Input: part model. Units: mm. Frame: model coordinates. Give positions to 0.01 mm unless a question says otherwise; leave off trailing zeros. Loops run counter-clockwise (first coordinate to the right, second up) from the corner with the lowest first, then second, coordinate; pieces in that order, holes last. Notation, with made-up numbers: M 3,-19 L 42,-19 A26 ccw 42,3 Z; hole C -4.75,67 d9. An arc over 180 degrees is marked long. Return JSON: item names as keys, results as strings. Group by question number.
```python
from build123d import *

# Parameters (mm, degrees)
SKETCH_1_R          = 2
EXTRUDE_1_DEPTH     = 4
CUT_EXTRUDE_1_DEPTH = 4
EXTRUDE_2_DEPTH     = 4
EXTRUDE_3_DEPTH     = 4
SKETCH_18_R         = 2
CUT_EXTRUDE_2_DEPTH = 5
CUT_EXTRUDE_3_DEPTH = 5


with BuildPart() as part:
    # 草图1 → 凸台-拉伸1 (new body)
    with BuildSketch(Plane.XY):
        with BuildLine():
            Line((153.5, -28), (-153.5, -28))
            ThreePointArc((-153.5, -28), (-156.328427125, -26.828427125), (-157.5, -24))
            Line((-157.5, -24), (-157.5, 24))
            ThreePointArc((-157.5, 24), (-156.328427125, 26.828427125), (-153.5, 28))
            Line((-153.5, 28), (153.5, 28))
            ThreePointArc((153.5, 28), (156.328427125, 26.828427125), (157.5, 24))
            Line((157.5, 24), (157.5, -24))
            ThreePointArc((157.5, -24), (156.328427125, -26.828427125), (153.5, -28))
        make_face()
        with Locations((-100, 23)):
            Circle(SKETCH_1_R, mode=Mode.SUBTRACT)
        with Locations((-61.67, 23)):
            Circle(SKETCH_1_R, mode=Mode.SUBTRACT)
        with Locations((-100, -23)):
            Circle(SKETCH_1_R, mode=Mode.SUBTRACT)
        with Locations((-61.67, -23)):
            Circle(SKETCH_1_R, mode=Mode.SUBTRACT)
        with Locations((100, -23)):
            Circle(SKETCH_1_R, mode=Mode.SUBTRACT)
        with Locations((61.67, -23)):
            Circle(SKETCH_1_R, mode=Mode.SUBTRACT)
        with Locations((61.67, 23)):
            Circle(SKETCH_1_R, mode=Mode.SUBTRACT)
        with Locations((100, 23)):
            Circle(SKETCH_1_R, mode=Mode.SUBTRACT)
        with BuildLine():
            Line((-150, -13.9), (-50, -13.9))
            ThreePointArc((-50, -13.9), (-47.9, -16), (-50, -18.1))
            Line((-50, -18.1), (-150, -18.1))
            ThreePointArc((-150, -18.1), (-152.1, -16), (-150, -13.9))
        make_face(mode=Mode.SUBTRACT)
    extrude(amount=EXTRUDE_1_DEPTH)

    # 草图2 → 切除-拉伸1 (cut)
    with BuildSketch(Plane.XY.offset(4)):
        with BuildLine():
            Line((0, -12), (0, -24))
            ThreePointArc((0, -24), (-1.171572875, -26.828427125), (-4, -28))
            Line((-4, -28), (0, -28))
            Line((0, -28), (157.5, -28))
            Line((157.5, -28), (157.5, -2))
            Line((157.5, -2), (157.5, 2))
            ThreePointArc((157.5, 2), (156.328427125, -0.828427125), (153.5, -2))
            Line((153.5, -2), (146.462792112, -2))
            Line((146.462792112, -2), (108, -2))
            Line((108, -2), (10, -2))
            ThreePointArc((10, -2), (2.928932188, -4.928932188), (0, -12))
        make_face()
    extrude(amount=-CUT_EXTRUDE_1_DEPTH, mode=Mode.SUBTRACT)

    # 草图3 → 凸台-拉伸2 (add)
    with BuildSketch(Plane.XY.offset(4)):
        with BuildLine():
            Line((-4, 28), (-4, -28))
            ThreePointArc((-4, -28), (-1.171572875, -26.828427125), (0, -24))
            Line((0, -24), (0, -12))
            ThreePointArc((0, -12), (2.928932188, -4.928932188), (10, -2))
            Line((10, -2), (26, -2))
            Line((26, -2), (26, 24))
            ThreePointArc((26, 24), (27.171572875, 26.828427125), (30, 28))
            Line((30, 28), (26, 28))
            Line((26, 28), (-4, 28))
        make_face()
        with BuildLine():
            ThreePointArc((0, -24), (-1.171572875, -26.828427125), (-4, -28))
            Line((-4, -28), (22, -28))
            ThreePointArc((22, -28), (24.828427125, -26.828427125), (26, -24))
            Line((26, -24), (26, -2))
            Line((26, -2), (10, -2))
            ThreePointArc((10, -2), (2.928932188, -4.928932188), (0, -12))
            Line((0, -12), (0, -24))
        make_face()
    extrude(amount=-EXTRUDE_2_DEPTH)

    # 草图17 → 凸台-拉伸3 (add)
    with BuildSketch(Plane.XY.offset(4)):
        with BuildLine():
            Line((26, -2), (26, -8.742458912))
            Line((26, -8.742458912), (26, -17))
            ThreePointArc((26, -17), (30.393398282, -6.393398282), (41, -2))
            Line((41, -2), (26, -2))
        make_face()
    extrude(amount=-EXTRUDE_3_DEPTH)

    # 草图18 → 切除-拉伸2 (cut, through all)
    with BuildSketch(Plane.XY.offset(4)):
        with Locations((0, -16)):
            Circle(SKETCH_18_R)
    extrude(amount=-CUT_EXTRUDE_2_DEPTH, mode=Mode.SUBTRACT)

    # 草图19 → 切除-拉伸3 (cut, through all)
    with BuildSketch(Plane.XY.offset(4)):
        with BuildLine():
            Line((-50, -10.6), (-150, -10.6))
            ThreePointArc((-150, -10.6), (-153.6, -7), (-150, -3.4))
            Line((-150, -3.4), (-50, -3.4))
            ThreePointArc((-50, -3.4), (-46.4, -7), (-50, -10.6))
        make_face()
    extrude(amount=-CUT_EXTRUDE_3_DEPTH, mode=Mode.SUBTRACT)


solid = part.part
```
Item 1: Section D-D, the plane x = 74.5. Return loops of the section in (y, z), then the cut area to 3 significant figures.
Item 2: Material intervals for line 1 (Y direction, x = -61.67, z = 0.9); line 2 (Y direction, x = -143, z = 2.9); line 3 (X direction, y = -15.5, z = 0.85), sorted ascending. Write a range as from..to.
Item 3: First-contact query: pin 1 Ø2 at (y, z) = (-21, 2) entering from +X; pin 2 Ø8 at (x, y) = (-124.5, 16.5) entering from -Z; pin 3 Ø1.5 at (y, z) = (-15, 0.5) entering from +X; pin 4 Ø2.5 at (x, y) = (-100, 23) entering from +Z. Flat tips, straight axial feed; report the tip coordinate or a pass-through.
Item 4: Section C-C, the plane y = -7. Return loops of the section in (x, z).
Item 5: Section A-A, the plane x = -114. Return loops of the section in (y, z), then the cut area to 3 significant figures.
Item 6: Section B-B, the plane z = 2.3. Give the number of separate pieces and of enclosed holes in the cut face, then the cut area to 3 significant figures.
Answer below:
{
 "1": {"outline": "M -2,0 L 28,0 L 28,4 L -2,4 Z", "area": "120 mm^2"},
 "2": {"line 1": "-28..-25, -21..-18.1, -13.9..-10.6, -3.4..21, 25..28", "line 2": "-28..-18.1, -13.9..-10.6, -3.4..28", "line 3": "-157.5..-152.04, -47.96..-1.94, 1.94..26.08"},
 "3": {"pin 1": "x = 26", "pin 2": "z = 0", "pin 3": "x = 26.25", "pin 4": "through"},
 "4": {"outline": "M -157.5,0 L -153.6,0 L -153.6,4 L -157.5,4 Z; M -46.4,0 L 29.82,0 L 29.82,4 L -46.4,4 Z"},
 "5": {"outline": "M -28,0 L -18.1,0 L -18.1,4 L -28,4 Z; M -13.9,0 L -10.6,0 L -10.6,4 L -13.9,4 Z; M -3.4,0 L 28,0 L 28,4 L -3.4,4 Z", "area": "178 mm^2"},
 "6": {"separate pieces": "1", "enclosed holes": "9", "area": "13,000 mm^2"}
}
